```python
from build123d import *
from build123d.topology import SkipClean

# Parameters (mm, degrees)
SKIZZE2_W                            = 99.9
SKIZZE2_H                            = 2.25
SKIZZE3_W                            = 20
SKIZZE3_H                            = 20
SKIZZE3_R                            = 7.75
AUFSATZ_LINEAR_AUSTRAGEN1_DEPTH      = 6
SKIZZE5_R                            = 1.7
SCHNITT_LINEAR_AUSTRAGEN1_DEPTH      = 4
SCHNITT_LINEAR_AUSTRAGEN2_DEPTH      = 101.896035601
SCHNITT_LINEAR_AUSTRAGEN4_DEPTH      = 3
SCHNITT_LINEAR_AUSTRAGEN4_DEPTH_BACK = 101.896035601
SKIZZE8_W                            = 20
SKIZZE8_H                            = 15.917157288
AUFSATZ_LINEAR_AUSTRAGEN2_REACH      = 61.61
AUFSATZ_LINEAR_AUSTRAGEN11_DEPTH     = 20
SKIZZE20_R                           = 7.75
SCHNITT_LINEAR_AUSTRAGEN7_DEPTH      = 103.000049029
AUFSATZ_LINEAR_START                 = -21
SKIZZE21_R                           = 4.5
AUFSATZ_LINEAR_AUSTRAGEN12_DEPTH     = 22
SKIZZE22_R                           = 2.5
SCHNITT_LINEAR_AUSTRAGEN8_DEPTH      = 104.86534552
AUFSATZ_LINEAR_START_2               = -9.539392014
AUFSATZ_LINEAR_AUSTRAGEN14_DEPTH     = 2.39358905
AUFSATZ_LINEAR_START_3               = -20.918031139
AUFSATZ_LINEAR_AUSTRAGEN15_OUTLINE_W = 4.519922446
AUFSATZ_LINEAR_AUSTRAGEN15_OUTLINE_H = 9
AUFSATZ_LINEAR_AUSTRAGEN15_DEPTH     = 16.398108693
AUFSATZ_LINEAR_START_4               = 5.480077554
AUFSATZ_LINEAR_AUSTRAGEN15_2_DEPTH   = 4.519922446
AUFSATZ_LINEAR_START_5               = -54.45
AUFSATZ_LINEAR_AUSTRAGEN15_3_DEPTH   = 9
SKIZZE26_R                           = 7.75
SCHNITT_LINEAR_AUSTRAGEN9_DEPTH      = 9


with BuildPart() as part:
    # Skizze2 → Rotation1 (revolve)
    with BuildSketch(Plane(origin=(0, 0, 0), x_dir=(0, 0, -1), z_dir=(1, 0, 0)), mode=Mode.PRIVATE) as rotation1_sk:
        with Locations((49.95, 8.875)):
            Rectangle(SKIZZE2_W, SKIZZE2_H)
    revolve(rotation1_sk.sketch.rotate(Axis((0, 0, -49.15), (0, 0, -1)), 180), axis=Axis((0, 0, -49.15), (0, 0, -1)))

    # Skizze3 → Aufsatz-Linear austragen1 (add)
    with BuildSketch(Plane.XY):
        Rectangle(SKIZZE3_W, SKIZZE3_H)
        with Locations(Location((0, 0, 0), (0, 0, 270))):
            Circle(SKIZZE3_R, mode=Mode.SUBTRACT)
    aufsatz_linear_austragen1 = extrude(amount=-AUFSATZ_LINEAR_AUSTRAGEN1_DEPTH)

    # Skizze5 → Schnitt-Linear austragen1 (cut)
    with BuildSketch(Plane.XY):
        with Locations((-7.352290732, 7.352290732)):
            Circle(SKIZZE5_R)
        with Locations(Location((-7.352290732, -7.352290732, 0), (0, 0, 180))):
            Circle(SKIZZE5_R)
        with Locations((7.352290732, -7.352290732)):
            Circle(SKIZZE5_R)
        with Locations(Location((7.352290732, 7.352290732, 0), (0, 0, 180))):
            Circle(SKIZZE5_R)
    schnitt_linear_austragen1 = extrude(amount=-SCHNITT_LINEAR_AUSTRAGEN1_DEPTH, mode=Mode.SUBTRACT)

    # Spiegeln1: Aufsatz-Linear austragen1, Schnitt-Linear austragen1 across plane
    add(aufsatz_linear_austragen1.mirror(Plane.XY.offset(-49.95)))
    add(schnitt_linear_austragen1.mirror(Plane.XY.offset(-49.95)), mode=Mode.SUBTRACT)

    # Skizze6 → Schnitt-Linear austragen2 (cut, through all)
    with BuildSketch(Plane.XY):
        with BuildLine():
            Line((-10, 7.352290732), (-10.707106781, 7.352290732))
            Line((-10.707106781, 7.352290732), (-10.707106781, 10.707106781))
            Line((-10.707106781, 10.707106781), (-7.352290732, 10.707106781))
            Line((-7.352290732, 10.707106781), (-7.352290732, 10))
            ThreePointArc((-7.352290732, 10), (-9.22450391, 9.22450391), (-10, 7.352290732))
        make_face()
        with BuildLine():
            Line((7.352290732, 10.707106781), (7.352290732, 10))
            ThreePointArc((7.352290732, 10), (9.22450391, 9.22450391), (10, 7.352290732))
            Line((10, 7.352290732), (10.707106781, 7.352290732))
            Line((10.707106781, 7.352290732), (10.707106781, 10.707106781))
            Line((10.707106781, 10.707106781), (7.352290732, 10.707106781))
        make_face()
        with BuildLine():
            Line((10, -7.352290732), (10.707106781, -7.352290732))
            Line((10.707106781, -7.352290732), (10.707106781, -10.707106781))
            Line((10.707106781, -10.707106781), (7.352290732, -10.707106781))
            Line((7.352290732, -10.707106781), (7.352290732, -10))
            ThreePointArc((7.352290732, -10), (9.22450391, -9.22450391), (10, -7.352290732))
        make_face()
        with BuildLine():
            Line((-7.352290732, -10.707106781), (-7.352290732, -10))
            ThreePointArc((-7.352290732, -10), (-9.22450391, -9.22450391), (-10, -7.352290732))
            Line((-10, -7.352290732), (-10.707106781, -7.352290732))
            Line((-10.707106781, -7.352290732), (-10.707106781, -10.707106781))
            Line((-10.707106781, -10.707106781), (-7.352290732, -10.707106781))
        make_face()
    extrude(amount=-SCHNITT_LINEAR_AUSTRAGEN2_DEPTH, mode=Mode.SUBTRACT)

    # Skizze8 → Schnitt-Linear austragen4 (cut, two sides: drawn at the far end of the back side and taken through both)
    with BuildSketch(Plane(origin=(0, 0, 0), x_dir=(1, 0, 0), z_dir=(0, 1, 0)).offset(-SCHNITT_LINEAR_AUSTRAGEN4_DEPTH_BACK)):
        with Locations((0, 49.95)):
            Rectangle(SKIZZE8_W, SKIZZE8_H)
    extrude(amount=SCHNITT_LINEAR_AUSTRAGEN4_DEPTH + SCHNITT_LINEAR_AUSTRAGEN4_DEPTH_BACK, mode=Mode.SUBTRACT)

    # Skizze9 → Aufsatz-Linear austragen2 (add, up to next)
    with BuildSketch(Plane(origin=(0, 0, -41.991421356), x_dir=(-1, 0, 0), z_dir=(0, 0, -1)), mode=Mode.PRIVATE) as aufsatz_linear_austragen2_sk1:
        with BuildLine():
            Line((-9.539392014, 3), (-7.145802964, 3))
            ThreePointArc((-7.145802964, 3), (-7.604679056, -1.493772558), (-5.480077554, -5.480077554))
            Line((-5.480077554, -5.480077554), (-7.071067812, -7.071067812))
            ThreePointArc((-7.071067812, -7.071067812), (-9.712540637, -2.380452557), (-9.539392014, 3))
        make_face()
    aufsatz_linear_austragen2_tool1 = extrude(aufsatz_linear_austragen2_sk1.sketch, amount=AUFSATZ_LINEAR_AUSTRAGEN2_REACH, mode=Mode.PRIVATE) - part.part
    add(aufsatz_linear_austragen2_tool1.solids().sort_by_distance((8.235697, -1.849559, -41.991421))[0])

    # Skizze19 → Aufsatz-Linear austragen11 (add, through all)
    with BuildSketch(Plane.ZY.offset(10)):
        with BuildLine():
            Line((-51.686004996, 17.65166071), (-93.9, 0))
            Line((-93.9, 0), (-80.939207809, 0))
            Line((-80.939207809, 0), (-53.883064142, 11.31344873))
            ThreePointArc((-53.883064142, 11.31344873), (-49.95, 9), (-46.016935858, 11.31344873))
            Line((-46.016935858, 11.31344873), (-18.960792191, 0))
            Line((-18.960792191, 0), (-6, 0))
            Line((-6, 0), (-48.213995004, 17.65166071))
            ThreePointArc((-48.213995004, 17.65166071), (-49.95, 18), (-51.686004996, 17.65166071))
        make_face()
    extrude(amount=-AUFSATZ_LINEAR_AUSTRAGEN11_DEPTH)

    # Skizze20 → Schnitt-Linear austragen7 (cut, through all)
    with SkipClean():  # the faces are left unmerged after this step: merging them gives an invalid solid
        with BuildSketch(Plane(origin=(0, 0, -99.9), x_dir=(-1, 0, 0), z_dir=(0, 0, -1))):
            with Locations(Location((0, 0, 0), (0, 0, 270))):
                Circle(SKIZZE20_R)
        extrude(amount=-SCHNITT_LINEAR_AUSTRAGEN7_DEPTH, mode=Mode.SUBTRACT)

    # Skizze21 → Aufsatz-Linear austragen12 (add)
    with SkipClean():  # the faces are left unmerged after this step: merging them gives an invalid solid
        with BuildSketch(Plane.ZY.offset(10).offset(AUFSATZ_LINEAR_START)):
            with Locations((-49.95, 13.5)):
                Circle(SKIZZE21_R)
        extrude(amount=AUFSATZ_LINEAR_AUSTRAGEN12_DEPTH)

    # Skizze22 → Schnitt-Linear austragen8 (cut, through all)
    with SkipClean():  # the faces are left unmerged after this step: merging them gives an invalid solid
        with BuildSketch(Plane(origin=(11, 0, 0), x_dir=(0, 0, -1), z_dir=(1, 0, 0))):
            with Locations((49.95, 13.5)):
                Circle(SKIZZE22_R)
        extrude(amount=-SCHNITT_LINEAR_AUSTRAGEN8_DEPTH, mode=Mode.SUBTRACT)

    # Aufsatz-Linear austragen14: read off the stored shape, not the designer's step
    # Aufsatz-Linear austragen14 outline → Aufsatz-Linear austragen14 (add)
    with SkipClean():  # the faces are left unmerged after this step: merging them gives an invalid solid
        with BuildSketch(Plane.YZ.offset(AUFSATZ_LINEAR_START_2)):
            with BuildLine():
                Line((11.31344873, -46.016935858), (11.076386129, -45.45))
                Line((11.076386129, -45.45), (3, -45.45))
                Line((3, -45.45), (3, -54.45))
                Line((3, -54.45), (11.076386129, -54.45))
                Line((11.076386129, -54.45), (11.31344873, -53.883064142))
                ThreePointArc((11.31344873, -53.883064142), (9, -49.95), (11.31344873, -46.016935858))
            make_face()
        extrude(amount=AUFSATZ_LINEAR_AUSTRAGEN14_DEPTH)

    # Aufsatz-Linear austragen15: read off the stored shape, not the designer's step
    # Aufsatz-Linear austragen15 outline → Aufsatz-Linear austragen15 (add)
    with SkipClean():  # the faces are left unmerged after this step: merging them gives an invalid solid
        with BuildSketch(Plane(origin=(0, -10, 0), x_dir=(-1, 0, 0), z_dir=(0, -1, 0)).offset(AUFSATZ_LINEAR_START_3)):
            with Locations((-7.740038777, 49.95)):
                Rectangle(AUFSATZ_LINEAR_AUSTRAGEN15_OUTLINE_W, AUFSATZ_LINEAR_AUSTRAGEN15_OUTLINE_H)
        extrude(amount=AUFSATZ_LINEAR_AUSTRAGEN15_DEPTH)

    # Aufsatz-Linear austragen15 2 outline → Aufsatz-Linear austragen15 2 (add)
    with SkipClean():  # the faces are left unmerged after this step: merging them gives an invalid solid
        with BuildSketch(Plane.YZ.offset(AUFSATZ_LINEAR_START_4)):
            with BuildLine():
                Line((11.076386129, -45.45), (10.918031139, -45.45))
                Line((10.918031139, -45.45), (10.918031139, -46.264428565))
                ThreePointArc((10.918031139, -46.264428565), (11.112530792, -46.135554984), (11.31344873, -46.016935858))
                Line((11.31344873, -46.016935858), (11.076386129, -45.45))
            make_face()
            with BuildLine():
                Line((10.918031139, -53.635571435), (10.918031139, -54.45))
                Line((10.918031139, -54.45), (11.076386129, -54.45))
                Line((11.076386129, -54.45), (11.31344873, -53.883064142))
                ThreePointArc((11.31344873, -53.883064142), (11.112530792, -53.764445016), (10.918031139, -53.635571435))
            make_face()
        extrude(amount=AUFSATZ_LINEAR_AUSTRAGEN15_2_DEPTH)

    # Aufsatz-Linear austragen15 3 outline → Aufsatz-Linear austragen15 3 (add)
    with SkipClean():  # the faces are left unmerged after this step: merging them gives an invalid solid
        with BuildSketch(Plane.XY.offset(AUFSATZ_LINEAR_START_5)):
            with BuildLine():
                Line((7.071067812, -7.071067812), (10, -10))
                Line((10, -10), (10, -5.480077554))
                Line((10, -5.480077554), (8.364732512, -5.480077554))
                ThreePointArc((8.364732512, -5.480077554), (7.75878827, -6.308819588), (7.071067812, -7.071067812))
            make_face()
        extrude(amount=AUFSATZ_LINEAR_AUSTRAGEN15_3_DEPTH)

    # Skizze26 → Schnitt-Linear austragen9 (cut)
    with BuildSketch(Plane.XY.offset(-45.45)):
        with Locations(Location((0, 0, 0), (0, 0, 270))):
            Circle(SKIZZE26_R)
        with BuildLine():
            Line((7.071067812, -7.071067812), (10, -10))
            Line((10, -10), (10, 0))
            ThreePointArc((10, 0), (9.238795325, -3.826834324), (7.071067812, -7.071067812))
        make_face()
    extrude(amount=-SCHNITT_LINEAR_AUSTRAGEN9_DEPTH, mode=Mode.SUBTRACT)


solid = part.part
```
Model file for the job. Use its own axes, mm. A direction names the side the tool comes from. Round coordinates to 2 decimals unless told otherwise and drop trailing zeros. Order: outer loops, then holes, each group sorted by start corner. A loop starts at its lowest first (then second) coordinate and runs counter-clockwise, first axis right, second up. Notation, with made-up numbers: (49.5, 67) -> (103.5, 67) arc R15 ccw to (103.5, 82) -> close; hole circle Ø2 at (58.25, 87.5). An arc over 180 degrees is marked (long way). Use one line per item in the form item = value.
Item 1: Cut at B-B, the plane y = 13.5. Write the cut outline in (x, z).
Returned:
outline = (-11, -54.45) -> (-10, -54.45) -> (-10, -61.61) -> (10, -61.61) -> (10, -54.45) -> (11, -54.45) -> (11, -52.45) -> (-11, -52.45) -> close; (-11, -47.45) -> (11, -47.45) -> (11, -45.45) -> (10, -45.45) -> (10, -38.29) -> (-10, -38.29) -> (-10, -45.45) -> (-11, -45.45) -> close
Item 2: Cut at D-D, the plane y = 2. Give the number of separate pieces and of enclosed holes in the cut face, and give its area (3 significant figures).
Returned:
separate_pieces = 3
enclosed_holes = 0
area = 442 mm^2
Item 3: Cut at A-A, the plane z = -49.95. Write the cut outline in (x, y), and give its area (3 significant figures).
Returned:
outline = (-11, 9) -> (-9.54, 9) -> (-9.54, 3) -> (-7.15, 3) arc R7.75 cw (long way) to (5.48, -5.48) -> (7.07, -7.07) arc R10 ccw to (10, 0) -> (10, 9) -> (11, 9) -> (11, 11) -> (-11, 11) -> close; (-11, 16) -> (11, 16) -> (11, 18) -> (-11, 18) -> close; hole (-7.15, 7) arc R10 cw to (-4.36, 9) -> (-7.15, 9) -> close; hole (4.36, 9) arc R10 cw to (5.48, 8.36) -> (5.48, 9) -> close
area = 176 mm^2
Item 4: Pull direction X, two halves, no side cores. Call faces 4 (the face through (-9.05, 7.43, -97.93)), 5 (the face through (-0.14, 12.625, -36.192)), 6 (the face through (7, -7, -4)), 7 (the face through (-10, 7, -71)): released by +X, released by -X, zero draft, split by the parting line, or undercut.
Returned:
face_4 = undercut
face_5 = zero draft
face_6 = undercut
face_7 = released by -X
Item 5: Flat gauge pins, fed straight in: pin 1 Ø10 at (x, z) = (-8.5, -56) entering from -Y; pin 2 Ø12 at (y, z) = (3.5, -76.5) entering from +X; pin 3 Ø1 at (x, y) = (-7, 14.5) entering from +Z. Where does each tip first touch, or does it go through?
Returned:
pin_1 = -9.22
pin_2 = 10
pin_3 = -39.48
Item 6: Drill centre lines: line 1 (Z direction, x = -8.5, y = 0); line 2 (X direction, y = -0.25, z = -17); line 3 (X direction, y = 5.5, z = -5). Where is each one in solid material? Low to high.
Returned:
line_1 = -99.9 to -57.91, -41.99 to 0
line_2 = -10 to -7.75, 7.75 to 10
line_3 = -10 to -5.46, 5.46 to 10
Item 7: Tool access for faces 1 (the face through (7, 7, -4)), 2 (the face through (9.204, 9.245, -96.858)), 3 (the face through (-8, -8, -6)): list every direction of +Z, -Z, +X, -X, +Y, -Y with a clear straight run to the whole face (end or side of a thin tool).
Returned:
face_1 = +Z
face_2 = -Z, +X, +Y
face_3 = -X, -Y
